Here's how the part is built. I have some questions about the finished solid (model axes, mm). Face numbers are marked on the shaded views. A direction names the side the tool comes from. Coordinates: 2 decimals unless noted, no trailing zeros. Write each loop counter-clockwise with the first axis right and the second up, starting at its lowest first coordinate (ties: lowest second). Pieces come first, ordered by that corner, then holes.
Item 1: For the marked faces 5 and 6, which set-ups out of +Z, -Z, +X, -X, +Y, -Y let a thin tool reach every point of the face, with its end or its side?
Item 2: I want a section at A-A (y = 26). Please give me the cut outline in (x, z), and give its area (3 significant figures).
Item 3: Please list where these lines run through material, in increasing order: line 1 (Y direction, x = 24, z = 17.25); line 2 (X direction, y = 23.5, z = 14); line 3 (Z direction, x = -38, y = 30).
Item 4: I want a section at C-C (z = 14). Please give me the cut outline in (x, y), and give its area (3 significant figures).
Item 5: I want a section at D-D (z = 1.5). Please give me the cut outline in (x, y), and give its area (3 significant figures).
Item 6: I'm going to push a flat-ended pin straight in: P1, Ø2, axis at x = 28.5, y = 7, coming from the +Z side. Where does the tip first touch, or does it pass through?
Item 7: I want a section at B-B (x = 3.5). Please give me the cut outline in (y, z), and give its area (3 significant figures).
Item 8: If we mould it in two halves opening along Y, with no side actions, what happens to the marked faces 1, 2, 3 and 4? For each: pulls with the +Y half, pulls with the -Y half, needs draft (parallel to the pull), parting line crosses it, or undercut.
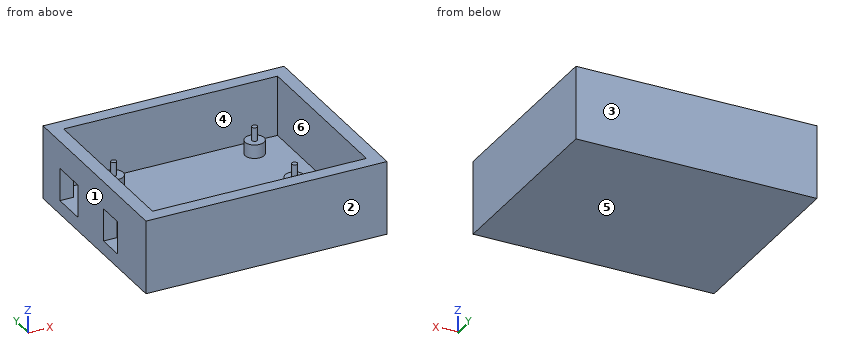
from build123d import *

# Parameters (mm, degrees)
F1_W          = 88.56
F1_H          = 73.2
F2_DEPTH      = 22
F2_DEPTH_BACK = 5
F3_W          = 78.56
F3_H          = 63.2
F4_DEPTH      = 34.1
F7_R          = 3.5
F7_R_2        = 1
F8_DEPTH      = 5
F6_W          = 13
F6_H          = 12
F6_W_2        = 10
F9_DEPTH      = 25
F10_R         = 1
F11_DEPTH     = 10


with BuildPart() as f2:
    # F1 (on Top) → F2 (new body, two sides)
    with BuildSketch(Plane.XY) as f2_sk:
        with Locations((1.572817, 11.100315)):
            Rectangle(F1_W, F1_H)
    extrude(amount=F2_DEPTH)
    extrude(f2_sk.sketch, amount=-F2_DEPTH_BACK)

    # F3 (on Top) → F4 (cut)
    with BuildSketch(Plane.XY):
        with Locations((1.572817, 11.100315)):
            Rectangle(F3_W, F3_H)
    extrude(amount=F4_DEPTH, mode=Mode.SUBTRACT)

    # F7 (on face) → F8 (join)
    with BuildSketch(Plane.XY):
        with Locations((28.572817, 35.200315)):
            Circle(F7_R)
        with Locations((28.572817, 35.200315)):
            Circle(F7_R_2, mode=Mode.SUBTRACT)
        with Locations((28.572817, 6.700315)):
            Circle(F7_R)
        with Locations((28.572817, 6.700315)):
            Circle(F7_R_2, mode=Mode.SUBTRACT)
        with Locations((-23.207183, 35.200315)):
            Circle(F7_R)
        with Locations((-23.207183, 35.200315)):
            Circle(F7_R_2, mode=Mode.SUBTRACT)
        with Locations((-23.207183, -12.999685)):
            Circle(F7_R)
        with Locations((-23.207183, -12.999685)):
            Circle(F7_R_2, mode=Mode.SUBTRACT)
    extrude(amount=F8_DEPTH)

    # F6 (on face) → F9 (cut)
    with BuildSketch(Plane.YZ.offset(-37.707183)):
        with Locations((29.200315, 6)):
            Rectangle(F6_W, F6_H)
        with Locations((-0.299685, 6)):
            Rectangle(F6_W_2, F6_H)
    extrude(amount=-F9_DEPTH, mode=Mode.SUBTRACT)

    # F10 (on face) → F11 (join)
    with BuildSketch(Plane.XY):
        with Locations((28.572817, 35.200315)):
            Circle(F10_R)
        with Locations((28.572817, 6.700315)):
            Circle(F10_R)
        with Locations((-23.207183, -12.999685)):
            Circle(F10_R)
        with Locations((-23.207183, 35.200315)):
            Circle(F10_R)
    extrude(amount=F11_DEPTH)


solid = f2.part
Answer:
1. face 5: -Z, +X, -X, +Y, -Y
1. face 6: +Z
2. outline: (-42.71, -5) - (45.85, -5) - (45.85, 22) - (40.85, 22) - (40.85, 0) - (-42.71, 0) - close; (-42.71, 12) - (-37.71, 12) - (-37.71, 22) - (-42.71, 22) - close
2. area: 603 mm2
3. line 1: y = -25.5 to -20.5, 42.7 to 47.7
3. line 2: x = -42.71 to -37.71, 40.85 to 45.85
3. line 3: z = -5 to 0, 12 to 22
4. outline: (-42.71, -25.5) - (45.85, -25.5) - (45.85, 47.7) - (-42.71, 47.7) - close; hole (-37.71, -20.5) - (40.85, -20.5) - (40.85, 42.7) - (-37.71, 42.7) - close
4. area: 1,520 mm2
5. outline: (-42.71, -25.5) - (45.85, -25.5) - (45.85, 47.7) - (-42.71, 47.7) - (-42.71, 35.7) - (-37.71, 35.7) - (-37.71, 42.7) - (40.85, 42.7) - (40.85, -20.5) - (-37.71, -20.5) - (-37.71, -5.3) - (-42.71, -5.3) - close; (-42.71, 4.7) - (-37.71, 4.7) - (-37.71, 22.7) - (-42.71, 22.7) - close; circle Ø7 at (-23.21, -13); circle Ø7 at (-23.21, 35.2); circle Ø7 at (28.57, 6.7); circle Ø7 at (28.57, 35.2)
5. area: 1,560 mm2
6. P1: stops at z = 10
7. outline: (-25.5, -5) - (47.7, -5) - (47.7, 22) - (42.7, 22) - (42.7, 0) - (-20.5, 0) - (-20.5, 22) - (-25.5, 22) - close
7. area: 586 mm2
8. face 1: needs draft
8. face 2: pulls with the -Y half
8. face 3: pulls with the +Y half
8. face 4: undercut
